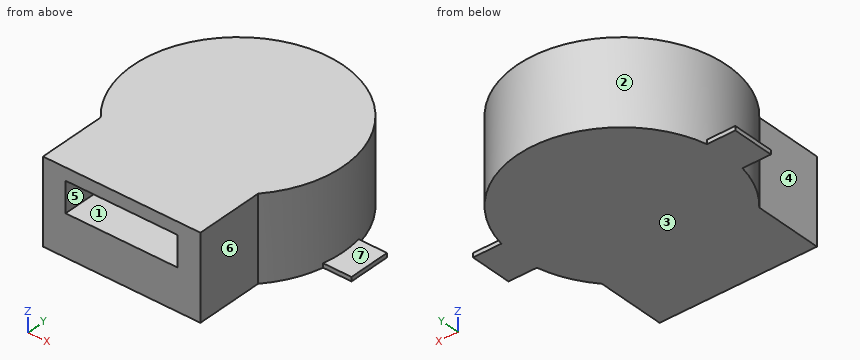
```python
from build123d import *

# Parameters (mm, degrees)
PAD_DEPTH    = 3.2
SKETCH001_W  = 1.6
SKETCH001_H  = 0.16
PAD001_DEPTH = 2
SKETCH002_W  = 4.264834
SKETCH002_H  = 1.156565
POCKET_DEPTH = 5


with BuildPart() as part:
    # Sketch → Pad (new body)
    with BuildSketch(Plane.XY):
        with BuildLine():
            ThreePointArc((3, -2.645751), (0, 4), (-3, -2.645751))
            Line((-3, -2.645751), (-3, -5.245751))
            Line((-3, -5.245751), (3, -5.245751))
            Line((3, -5.245751), (3, -2.645751))
        make_face()
    extrude(amount=PAD_DEPTH)

    # Sketch001 (on Face2 of Pad) → Pad001 (join)
    with BuildSketch(Plane(origin=(-3, 0, 0), x_dir=(0, -1, 0), z_dir=(-1, 0, 0))):
        with Locations((0, 0.08)):
            Rectangle(SKETCH001_W, SKETCH001_H)
    pad001 = extrude(amount=PAD001_DEPTH)

    # Mirrored: Pad001 across YZ
    add(pad001.mirror(Plane.YZ))

    # Sketch002 (on Face12 of Mirrored) → Pocket (cut)
    with BuildSketch(Plane.XZ.offset(5.245751)):
        with Locations((-0.006884, 2.148988)):
            Rectangle(SKETCH002_W, SKETCH002_H)
    extrude(amount=-POCKET_DEPTH, mode=Mode.SUBTRACT)


solid = part.part
```
The listing builds one solid part. Answer for the finished solid, in the listing's coordinates (mm). Face numbers are marked on the shaded views. A direction names the side the tool comes from. Give positions to 0.01 mm unless a question says otherwise; leave off trailing zeros. Order: outer loops, then holes, each group sorted by start corner. A loop starts at its lowest first (then second) coordinate and runs counter-clockwise, first axis right, second up. Notation, with made-up numbers: (-13.5, 74.25) - (-2.5, 74.25) arc R29 cw to (-2.5, 104.25) - close; hole circle Ø3 at (57, 30.5). An arc over 180 degrees is marked (long way). Answer in a Markdown table with one row per item. Add a question column.
Q1. Find the intervals of material crossed by line 1 along Z through (x, y) = (-2, -4.75); line 2 along X through (y, z) = (-3.5, 1.8); line 3 along X through (y, z) = (-3.25, 1), in increasing order. Write a range as [from, to].
Q2. For a pull along Z with two mould halves and no side action, classify the marked faces 5, 6 and 7 as released by +Z, released by -Z, zero draft, split by the parting line, or undercut.
Q3. The part is cut by section C-C (y = -3.5). Determine the outline of the cut face in (x, z).
Q4. Which of the six approach directions +Z, -Z, +X, -X, +Y, -Y give full straight-line access (tool end or side, diameter ignored) to the marked faces 1, 2, 3 and 4?
Q5. Given P1, Ø1, axis at y = 1.5, z = 2, coming from the +X side; P2, Ø0.6, axis at y = -4, z = 2, coming from the -X side, each flat-ended and moving along its own axis, determine where each tip first touches the part or whether it passes through.
Q6. The part is cut by section B-B (y = 0). Determine the outline of the cut face in (x, z).
Q7. The part is cut by section A-A (z = 2). Determine the outline of the cut face in (x, y).
Q8. The part is cut by section D-D (x = -3.5). Determine the outline of the cut face in (y, z).
Determined:
| question | item | result |
|---|---|---|
| 1 | line 1 | z = [0, 1.57], [2.73, 3.2] |
| 1 | line 2 | x = [-3, -2.14], [2.13, 3] |
| 1 | line 3 | x = [-3, 3] |
| 2 | face 5 | undercut |
| 2 | face 6 | zero draft |
| 2 | face 7 | released by +Z |
| 3 | outline | (-3, 0) - (3, 0) - (3, 3.2) - (-3, 3.2) - close; hole (-2.14, 1.57) - (2.13, 1.57) - (2.13, 2.73) - (-2.14, 2.73) - close |
| 4 | face 1 | -Y |
| 4 | face 2 | +Z |
| 4 | face 3 | -Z, +X, -X, +Y, -Y |
| 4 | face 4 | +Z, -Z, -X, -Y |
| 5 | P1 | stops at x = 3.87 |
| 5 | P2 | stops at x = -3 |
| 6 | outline | (-5, 0) - (5, 0) - (5, 0.16) - (4, 0.16) - (4, 3.2) - (-4, 3.2) - (-4, 0.16) - (-5, 0.16) - close |
| 7 | outline | (-3, -5.25) - (-2.14, -5.25) - (-2.14, -0.25) - (2.13, -0.25) - (2.13, -5.25) - (3, -5.25) - (3, -2.65) arc R4 ccw (long way) to (-3, -2.65) - close |
| 8 | outline | (-1.94, 0) - (1.94, 0) - (1.94, 3.2) - (-1.94, 3.2) - close |
